Design review of the part built by this model. Coordinates are the model's own, in mm. A direction names the side the tool comes from. Round coordinates to 2 decimals unless told otherwise and drop trailing zeros. Loops run counter-clockwise (first coordinate to the right, second up) from the corner with the lowest first, then second, coordinate; pieces in that order, holes last. Notation, with made-up numbers: (-21.5, 37.5) - (-15.5, 37.5) arc R24 ccw to (-15.5, 62.5) - close; hole circle Ø7 at (9.5, -0.75). An arc over 180 degrees is marked (long way). Return JSON: item names as keys, results as strings. Group by question number.
(1) The part is to be moulded in two halves that separate along X. For faces 3 (the cylindrical face through (5.948, -5.07, 1.228)), 4 (the flat face through (0, -5, 25)), 5 (the flat face through (20, -5, 0)), say which applies: pulls with the +X half, pulls with the -X half, needs draft (parallel to the pull), parting line crosses it, or undercut.
(2) For faces 1 (the cylindrical face through (13.56, -5.07, 12.83)), 2 (the flat face through (20, -10, 31)), list the 3-axis set-ups (+Z, -Z, +X, -X, +Y, -Y) from which the entire face can be reached by the end or side of a thin tool; tool diameter is ignored.
(3) We need section A-A, the plane y = -1.5. Write out the cut boundary in (x, z), and give its area (3 significant figures).
(4) We need section C-C, the plane x = 17. Write out the cut boundary in (y, z).
(5) Clearance check with a flat-ended pin moving along its axis: pin 1 (3 mm diameter, centred on x = 9.5, z = 19.5, fed in from +Y). State where the tip first meets the part, or that it passes through.
(6) Wall thickness on L1, parallel to X at y = -6.75, z = 33; L2, parallel to X at y = -3, z = 5; L3, parallel to Z at x = 6.5, y = -9: over which ranges is each line inside the solid? List them lowest first. Write a range as [from, to].
(7) We need section B-B, the plane z = 20. Write out the cut boundary in (x, y).
from build123d import *

# Parameters (mm, degrees)
F0_W     = 40
F0_H     = 50
F1_DEPTH = 10
F3_DEPTH = 10.001


with BuildPart() as f1:
    # F0 (on Front) → F1 (new body)
    with BuildSketch(Plane.XZ):
        with Locations((20, 25)):
            Rectangle(F0_W, F0_H)
    extrude(amount=F1_DEPTH)

    # F2 (on face) → F3 (cut, through all)
    with BuildSketch(Plane.XZ.offset(10)):
        with BuildLine():
            Line((3.017207, 12.76887), (2, 7))
            ThreePointArc((2, 7), (6.055798, 1.20772), (11.848078, 5.263518))
            Line((11.848078, 5.263518), (12.865285, 11.032388))
            ThreePointArc((12.865285, 11.032388), (13.572367, 12.850646), (14.921442, 14.259908))
            Line((14.921442, 14.259908), (26.670659, 22.486798))
            ThreePointArc((26.670659, 22.486798), (30.717884, 26.714585), (32.839129, 32.169356))
            Line((32.839129, 32.169356), (33.856336, 37.938226))
            ThreePointArc((33.856336, 37.938226), (29.800538, 43.730506), (24.008258, 39.674708))
            Line((24.008258, 39.674708), (22.991051, 33.905838))
            ThreePointArc((22.991051, 33.905838), (22.283969, 32.087581), (20.934894, 30.678319))
            Line((20.934894, 30.678319), (9.185677, 22.451428))
            ThreePointArc((9.185677, 22.451428), (5.138452, 18.223642), (3.017207, 12.76887))
        make_face()
    extrude(amount=-F3_DEPTH, mode=Mode.SUBTRACT)


solid = f1.part
Solutions:
{
 "1": {"face 3": "undercut", "face 4": "pulls with the -X half", "face 5": "needs draft"},
 "2": {"face 1": "+Y, -Y", "face 2": "+Z, -Z, +X, -X, -Y"},
 "3": {"outline": "(0, 0) - (40, 0) - (40, 50) - (0, 50) - close; hole (2, 7) arc R5 ccw to (11.85, 5.26) - (12.87, 11.03) arc R5 cw to (14.92, 14.26) - (26.67, 22.49) arc R15 ccw to (32.84, 32.17) - (33.86, 37.94) arc R5 ccw to (24.01, 39.67) - (22.99, 33.91) arc R5 cw to (20.93, 30.68) - (9.19, 22.45) arc R15 ccw to (3.02, 12.77) - close", "area": "1,500 mm^2"},
 "4": {"outline": "(-10, 0) - (0, 0) - (0, 15.72) - (-10, 15.72) - close; (-10, 27.92) - (0, 27.92) - (0, 50) - (-10, 50) - close"},
 "5": {"pin 1": "through"},
 "6": {"L1": "[0, 22.74], [32.99, 40]", "L2": "[0, 2.05], [11.79, 40]", "L3": "[0, 1.15], [20.04, 50]"},
 "7": {"outline": "(0, -10) - (6.46, -10) - (6.46, 0) - (0, 0) - close; (23.12, -10) - (40, -10) - (40, 0) - (23.12, 0) - close"}
}
